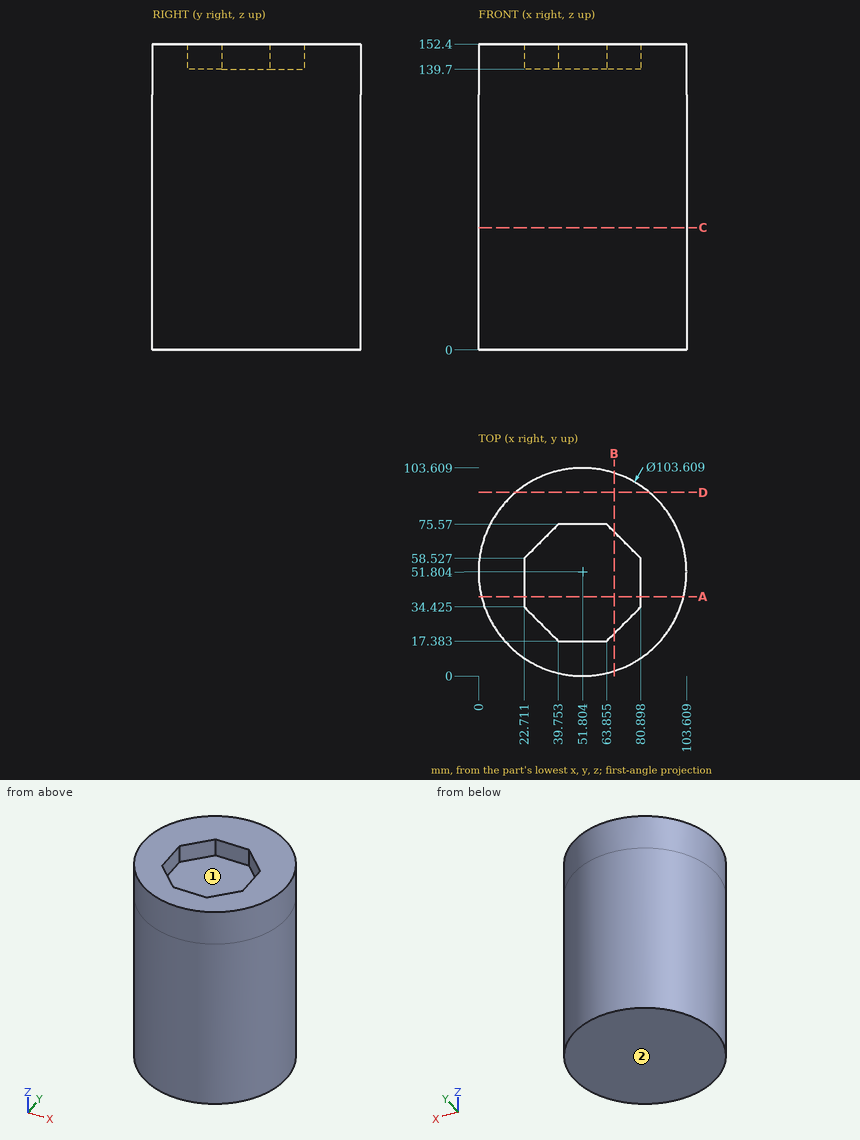
Verification items for this drawing (mm, ordinates from the low corner). Round coordinates to 2 decimals unless told otherwise and drop trailing zeros. Order: outer loops, then holes, each group sorted by start corner. A loop starts at its lowest first (then second) coordinate and runs counter-clockwise, first axis right, second up. Notation, with made-up numbers: (25.5, 79.5) - (69.5, 79.5) arc R28 ccw to (69.5, 97.5) - close; hole circle Ø1 at (16, 14.5). An arc over 180 degrees is marked (long way). Answer as CSV lines item,"result". Start each with the question number.
1) Section check C-C (z = 61). Record the cut outline in (x, y) (1 decimal), then the cut area to 3 significant figures.
2) Section check A-A (y = 39.5). Record the cut outline in (x, z), then the cut area to 3 significant figures.
3) Depth check by flat-ended pin: pin 1 (12 mm diameter, centred on x = 73, z = 51, fed in from +Y); pin 2 (4 mm diameter, centred on y = 43.5, z = 148, fed in from +X); pin 3 (4 mm diameter, centred on x = 56, z = 146, fed in from +Y). Enter the tip coordinate at first touch or a pass-through.
4) Section check D-D (y = 91.5). Record the cut outline in (x, z), then the cut area to 3 significant figures.
5) Section check B-B (x = 67.5). Record the cut outline in (y, z) (1 decimal), then the cut area to 3 significant figures.
6) Draft check along X on the marked faces 1 and 2. Enter one of: +X half, -X half, draft (parallel to the pull), parting line (faces both ways), or undercut.
7) Scan lines: probe 1 along Z at (x, y) = (44.5, 51); probe 2 along X at (y, z) = (75.5, 25.5); probe 3 along Y at (x, z) = (55, 83.5). Record each from-to range of solid material in increasing order.
Determined:
1,outline,"circle Ø103.6 at (51.8, 51.8)"
1,area,"8,430 mm^2"
2,outline,"(1.48, 0) - (102.13, 0) - (102.13, 152.4) - (80.9, 152.4) - (80.9, 139.7) - (22.71, 139.7) - (22.71, 152.4) - (1.48, 152.4) - close"
2,area,"14,600 mm^2"
3,pin 1,"y = 101.33"
3,pin 2,"x = 103.22"
3,pin 3,"y = 103.56"
4,outline,"(18.52, 0) - (85.09, 0) - (85.09, 152.4) - (18.52, 152.4) - close"
4,area,"10,100 mm^2"
5,outline,"(2.4, 0) - (101.2, 0) - (101.2, 152.4) - (71.9, 152.4) - (71.9, 139.7) - (21, 139.7) - (21, 152.4) - (2.4, 152.4) - close"
5,area,"14,400 mm^2"
6,face 1,"undercut"
6,face 2,"draft"
7,probe 1,"0 to 139.7"
7,probe 2,"5.74 to 97.87"
7,probe 3,"0.1 to 103.51"
